from build123d import *

# Parameters (mm, degrees)
SKETCH_1_R               = 20
EXTRUDE_1_DEPTH          = 29.5
CUT_EXTRUDE_1_DEPTH      = 30
CUT_EXTRUDE_1_DEPTH_BACK = 30
SKETCH_2_W               = 26.4
SKETCH_2_H               = 13.2
SKETCH_4_R               = 1.7
CUT_EXTRUDE_3_DEPTH      = 41.868692174
SKETCH_5_R               = 12.5
EXTRUDE_2_DEPTH          = 20
SKETCH_6_R               = 9.8
EXTRUDE_3_DEPTH          = 7
CUT_EXTRUDE_7_REACH      = 65.184
SKETCH_7_R               = 2.2
CUT_EXTRUDE_8_DEPTH      = 49.70821286
CUT_EXTRUDE_8_DEPTH_BACK = 49.70821286
SKETCH_8_R               = 2.2
CUT_EXTRUDE_START        = -5
SKETCH_9_R               = 3.75
CUT_EXTRUDE_9_DEPTH      = 10
CUT_EXTRUDE_START_2      = 41
SKETCH_10_R              = 3.75
CUT_EXTRUDE_10_DEPTH     = 10
FILLET_1_R               = 0.5
FILLET_2_R               = 1


with BuildPart() as part:
    # Sketch 1 → Extrude 1 (new body)
    with BuildSketch(Plane.XY):
        Circle(SKETCH_1_R)
    extrude(amount=EXTRUDE_1_DEPTH)

    # Sketch 2 → Cut-Extrude 1 (cut, two sides: drawn at the far end of the back side and taken through both)
    with BuildSketch(Plane(origin=(0, 0, 0), x_dir=(1, 0, 0), z_dir=(0, 1, 0)).offset(-CUT_EXTRUDE_1_DEPTH_BACK)):
        with Locations((0, -14.8)):
            Rectangle(SKETCH_2_W, SKETCH_2_H)
    extrude(amount=CUT_EXTRUDE_1_DEPTH + CUT_EXTRUDE_1_DEPTH_BACK, mode=Mode.SUBTRACT)

    # Sketch 4 → Cut-Extrude 3 (cut, through all)
    with BuildSketch(Plane(origin=(0, 0, 0), x_dir=(-1, 0, 0), z_dir=(0, 0, -1))):
        with Locations((0, 16)):
            Circle(SKETCH_4_R)
        with Locations((16, 0)):
            Circle(SKETCH_4_R)
        with Locations((0, -16)):
            Circle(SKETCH_4_R)
        with Locations((-16, 0)):
            Circle(SKETCH_4_R)
    extrude(amount=-CUT_EXTRUDE_3_DEPTH, mode=Mode.SUBTRACT)

    # Sketch 5 → Extrude 2 (add)
    with BuildSketch(Plane(origin=(0, 0, 0), x_dir=(-1, 0, 0), z_dir=(0, 0, -1))):
        with Locations(Location((0, 0, 0), (0, 0, 180))):
            Circle(SKETCH_5_R)
    extrude(amount=EXTRUDE_2_DEPTH)

    # Sketch 6 → Extrude 3 (add)
    with BuildSketch(Plane(origin=(0, 0, -20), x_dir=(-1, 0, 0), z_dir=(0, 0, -1))):
        Circle(SKETCH_6_R)
    extrude(amount=EXTRUDE_3_DEPTH)

    # Sketch 7 → Cut-Extrude 7 (cut, up to next)
    with BuildSketch(Plane(origin=(0, 0, -27), x_dir=(-1, 0, 0), z_dir=(0, 0, -1)), mode=Mode.PRIVATE) as cut_extrude_7_sk1:
        with Locations((0, 6.2)):
            Circle(SKETCH_7_R)
    cut_extrude_7_tool1 = extrude(cut_extrude_7_sk1.sketch, amount=-CUT_EXTRUDE_7_REACH, mode=Mode.PRIVATE) & part.part
    # Sketch 7 → Cut-Extrude 7 (cut, up to next)
    with BuildSketch(Plane(origin=(0, 0, -27), x_dir=(-1, 0, 0), z_dir=(0, 0, -1)), mode=Mode.PRIVATE) as cut_extrude_7_sk2:
        with Locations((0, -6.2)):
            Circle(SKETCH_7_R)
    cut_extrude_7_tool2 = extrude(cut_extrude_7_sk2.sketch, amount=-CUT_EXTRUDE_7_REACH, mode=Mode.PRIVATE) & part.part
    add(cut_extrude_7_tool1.solids().sort_by_distance((0, 6.2, -27))[0], mode=Mode.SUBTRACT)
    add(cut_extrude_7_tool2.solids().sort_by_distance((0, -6.2, -27))[0], mode=Mode.SUBTRACT)

    # Sketch 8 → Cut-Extrude 8 (cut, two sides: drawn at the far end of the back side and taken through both)
    with BuildSketch(Plane(origin=(-13.2, 0, 0), x_dir=(0, 0, -1), z_dir=(1, 0, 0)).offset(-CUT_EXTRUDE_8_DEPTH_BACK)):
        with Locations((-14.8, 6.2)):
            Circle(SKETCH_8_R)
        with Locations((-14.8, -6.2)):
            Circle(SKETCH_8_R)
    extrude(amount=CUT_EXTRUDE_8_DEPTH + CUT_EXTRUDE_8_DEPTH_BACK, mode=Mode.SUBTRACT)

    # Sketch 9 → Cut-Extrude 9 (cut)
    with BuildSketch(Plane(origin=(-13.2, 0, 0), x_dir=(0, 0, -1), z_dir=(1, 0, 0)).offset(CUT_EXTRUDE_START)):
        with Locations((-14.8, 6.2)):
            Circle(SKETCH_9_R)
        with Locations((-14.8, -6.2)):
            Circle(SKETCH_9_R)
    extrude(amount=-CUT_EXTRUDE_9_DEPTH, mode=Mode.SUBTRACT)

    # Sketch 10 → Cut-Extrude 10 (cut)
    with BuildSketch(Plane(origin=(-13.2, 0, 0), x_dir=(0, 0, -1), z_dir=(1, 0, 0)).offset(CUT_EXTRUDE_START_2)):
        with Locations((-14.8, 6.2)):
            Circle(SKETCH_10_R)
        with Locations((-14.8, -6.2)):
            Circle(SKETCH_10_R)
    extrude(amount=-CUT_EXTRUDE_10_DEPTH, mode=Mode.SUBTRACT)

    # Fillet 1
    fillet_1_edges = [part.edges().sort_by_distance(p)[0] for p in [
        (-20, 0, 0),
        (-12.5, 0, -20),
        (9.8, 0, -27),
    ]]
    fillet(fillet_1_edges, radius=FILLET_1_R)

    # Fillet 2
    fillet_2_edges = [part.edges().sort_by_distance(p)[0] for p in [
        (-12.5, 0, 0),
    ]]
    fillet(fillet_2_edges, radius=FILLET_2_R)


solid = part.part
Part model, mm, in its own coordinate system. A direction names the side the tool comes from. Coordinates: 2 decimals unless noted, no trailing zeros. Use a Markdown table: item, result.
(1) Flat gauge pins, fed straight in: pin 1 (5.5 mm diameter, centred on y = -6.2, z = 14.8, fed in from +X); pin 2 (3 mm diameter, centred on y = -5, z = 14.5, fed in from -X); pin 3 (4 mm diameter, centred on y = -6.2, z = 14.8, fed in from -X); pin 4 (3 mm diameter, centred on y = 16, z = -1, fed in from -X). Where does each tip first touch, or does it go through?
A:
| item | result |
|---|---|
| pin 1 | stops at x = 17.8 |
| pin 2 | stops at x = -18.2 |
| pin 3 | passes through |
| pin 4 | stops at x = -12.97 |
(2) Cut at A-A on z = 14.8. State how many separate pieces and enclosed holes the cut face has, then the cut area to 3 significant figures.
A:
| item | result |
|---|---|
| separate pieces | 6 |
| enclosed holes | 2 |
| area | 153 mm^2 |
(3) Probe L1, parallel to Y at x = 0, z = 23; L2, parallel to Z at x = -12.5, y = -12.5; L3, parallel to Y at x = 2, z = 4. List the from-to ranges inside material, lowest first.
A:
| item | result |
|---|---|
| L1 | y = -20 to -17.7, -14.3 to 14.3, 17.7 to 20 |
| L2 | z = 0 to 8.2, 21.4 to 29.5 |
| L3 | y = -19.9 to -7.12, -5.28 to 5.28, 7.12 to 19.9 |
(4) Pull direction X, two halves, no side cores. Call faces 4 (the cylindrical face through (0, -4, -10)), 5 (the cylindrical face through (-19.98, 0.88, 14.8)), 6 (the flat face through (0, 0, 29.5)), 7 (the flat face through (17.8, -4, 13)): released by +X, released by -X, zero draft, split by the parting line, or undercut.
A:
| item | result |
|---|---|
| face 4 | undercut |
| face 5 | split by the parting line |
| face 6 | zero draft |
| face 7 | released by +X |
(5) Tool access for faces 1 (the flat face through (-5, -13, 0)), 2 (the flat face through (-18.2, 4, 16)), 3 (the flat face through (0, 0, -27)): list every direction of +Z, -Z, +X, -X, +Y, -Y with a clear straight run to the whole face (end or side of a thin tool).
A:
| item | result |
|---|---|
| face 1 | -Z |
| face 2 | -X |
| face 3 | -Z, +X, -X, +Y, -Y |
